Model file for the job. Use its own axes, mm. Face numbers are marked on the shaded views. A direction names the side the tool comes from. Coordinates: 2 decimals unless noted, no trailing zeros. Order: outer loops, then holes, each group sorted by start corner. A loop starts at its lowest first (then second) coordinate and runs counter-clockwise, first axis right, second up. Notation, with made-up numbers: (-11.5, -19.5) - (42.5, -19.5) arc R25 ccw to (42.5, 17.5) - close; hole circle Ø10 at (73.5, 64.5). An arc over 180 degrees is marked (long way). Put each result on its own line as item: value. Start each with the question number.
```python
from build123d import *
from build123d.topology import SkipClean

# Parameters (mm, degrees)
SKETCH_1_W                = 76.6
SKETCH_1_H                = 23.8
EXTRUDE_1_DEPTH           = 31.899999991
HOLE_WIZARD_M4_1_D        = 3.3
HOLE_WIZARD_M4_1_DEPTH    = 10.1
HOLE_WIZARD_M4_1_TIP      = 0.991420021
SKETCH_5_W                = 23.8
SKETCH_5_H                = 2.281370048
EXTRUDE_2_DEPTH           = 2.994
SKETCH_6_W                = 76.6
SKETCH_6_H                = 2.281370048
EXTRUDE_3_DEPTH           = 2.944
CUT_EXTRUDE_START         = -2.994
SKETCH_7_W                = 26.992148155
SKETCH_7_H                = 47.339562986
CUT_EXTRUDE_1_DEPTH       = 2.994
EXTRUDE_4_DEPTH           = 10
HOLE_WIZARD_3_D           = 6.6
HOLE_WIZARD_3_CBORE_D     = 11
HOLE_WIZARD_3_CBORE_DEPTH = 6.8
SKETCH_21_R               = 3.3
CUT_EXTRUDE_6_DEPTH       = 67.034934903
MM_2_D                    = 4
MM_2_DEPTH                = 5
MM_2_TIP                  = 1.201721238
CUT_EXTRUDE_7_DEPTH       = 5
SKETCH_26_W               = 46.053862543
SKETCH_26_H               = 10
CUT_EXTRUDE_8_DEPTH       = 76.924939501
CUT_EXTRUDE_9_DEPTH       = 67.034934903
SKETCH_29_R               = 1
CUT_EXTRUDE_10_DEPTH      = 2.281370048
EXTRUDE_START             = 4
EXTRUDE_5_DEPTH           = 4
CUT_EXTRUDE_11_DEPTH      = 0.5
EXTRUDE_6_DEPTH           = 0.499988059
CUT_EXTRUDE_12_DEPTH      = 28.181370038
SKETCH_35_W               = 0.334557313
SKETCH_35_H               = 10
CUT_EXTRUDE_13_DEPTH      = 100.522674932
CHAMFER_1_SIZE            = 2
HOLE_WIZARD_4_D           = 4.5
HOLE_WIZARD_4_CBORE_D     = 8
HOLE_WIZARD_4_CBORE_DEPTH = 25
CUT_EXTRUDE_14_DEPTH      = 67.269104052
CUT_EXTRUDE_15_DEPTH      = 6.281370048
EXTRUDE_9_DEPTH           = 0.006


with BuildPart() as part:
    # 草图1 → 凸台-拉伸1 (new body)
    with BuildSketch(Plane(origin=(0, 0, 0), x_dir=(1, 0, 0), z_dir=(0, 1, 0))):
        Rectangle(SKETCH_1_W, SKETCH_1_H)
    extrude(amount=-EXTRUDE_1_DEPTH)

    # M4 螺纹孔1
    with Locations(Plane(origin=(0, 0, -5.4), x_dir=(0, 0, 1), z_dir=(0, 1, 0))):
        with Locations((0, 0)):
            Hole(HOLE_WIZARD_M4_1_D / 2, depth=HOLE_WIZARD_M4_1_DEPTH)
            with Locations((0, 0, -(HOLE_WIZARD_M4_1_DEPTH + HOLE_WIZARD_M4_1_TIP / 2))):  # 118° drill point
                Cone(0, HOLE_WIZARD_M4_1_D / 2, HOLE_WIZARD_M4_1_TIP, mode=Mode.SUBTRACT)

    # 草图5 → 凸台-拉伸2 (add)
    with BuildSketch(Plane.ZY.offset(38.3)):
        with Locations((0, 1.140685024)):
            Rectangle(SKETCH_5_W, SKETCH_5_H)
    extrude(amount=-EXTRUDE_2_DEPTH)

    # 草图6 → 凸台-拉伸3 (add)
    with BuildSketch(Plane(origin=(0, 0, -11.9), x_dir=(-1, 0, 0), z_dir=(0, 0, -1))):
        with Locations((0, 1.140685024)):
            Rectangle(SKETCH_6_W, SKETCH_6_H)
    extrude(amount=-EXTRUDE_3_DEPTH)

    # 草图7 → 切除-拉伸1 (cut)
    with BuildSketch(Plane(origin=(38.3, 0, 0), x_dir=(0, 0, -1), z_dir=(1, 0, 0)).offset(CUT_EXTRUDE_START)):
        with Locations((-1.596074077, -8.230218498)):
            Rectangle(SKETCH_7_W, SKETCH_7_H)
    extrude(amount=CUT_EXTRUDE_1_DEPTH, mode=Mode.SUBTRACT)

    # 草图9 → 大小mm 暗销孔1 (revolve, cut)
    with BuildSketch(Plane(origin=(17.4625, 0, -4.384), x_dir=(0, 0, 1), z_dir=(1, 0, 0))):
        Polygon((0, 0), (0, 5.96137699), (1.6, 5), (1.6, 0), align=None)
    mm_1 = revolve(axis=Axis((17.4625, 6.35, -4.384), (0, -1, 0)), mode=Mode.SUBTRACT)

    # 镜向3: 大小mm 暗销孔1 across plane
    add(mm_1.mirror(Plane(origin=(0, 0, 0), x_dir=(0, 0, 1), z_dir=(1, 0, 0))), mode=Mode.SUBTRACT)

    # 草图16 → 凸台-拉伸4 (add)
    with BuildSketch(Plane.XZ.offset(31.899999991)):
        Polygon((-38.3, 6.921881597), (-55.247298311, -11.9), (-38.3, -11.9), align=None)
        Polygon((-33.817682057, 11.9), (-20.311621392, 26.9), (35.306, 26.9), (35.306, 11.9), align=None)
    extrude(amount=-EXTRUDE_4_DEPTH)

    # 打孔尺寸(%根据)内六角圆柱头螺钉的类型3 (through all)
    with Locations(Plane(origin=(-14.255841028, -21.899999991, 19.4), x_dir=(1, 0, 0), z_dir=(0, 1, 0))):
        with Locations((0, 0), (15, 0), (35, 0)):
            CounterBoreHole(HOLE_WIZARD_3_D / 2, HOLE_WIZARD_3_CBORE_D / 2, HOLE_WIZARD_3_CBORE_DEPTH)

    # 草图21 → 切除-拉伸6 (cut, through all)
    with BuildSketch(Plane(origin=(0, -21.899999991, 0), x_dir=(1, 0, 0), z_dir=(0, 1, 0))):
        with Locations(Location((-44.3, 5.9, 0), (0, 0, 180))):
            Circle(SKETCH_21_R)
    extrude(amount=-CUT_EXTRUDE_6_DEPTH, mode=Mode.SUBTRACT)

    # 大小mm 暗销孔2
    with Locations(Plane(origin=(10.744158972, -31.899999991, 9.4), x_dir=(0, 0, -1), z_dir=(0, -1, 0))):
        with Locations((0, 0)):
            Hole(MM_2_D / 2, depth=MM_2_DEPTH)
            with Locations((0, 0, -(MM_2_DEPTH + MM_2_TIP / 2))):  # 118° drill point
                Cone(0, MM_2_D / 2, MM_2_TIP, mode=Mode.SUBTRACT)

    # 草图25 → 切除-拉伸7 (cut)
    with BuildSketch(Plane.XZ.offset(31.899999991)):
        with BuildLine():
            Line((-9.755841028, 11.4), (-8.755841028, 11.4))
            ThreePointArc((-8.755841028, 11.4), (-6.755841028, 9.4), (-8.755841028, 7.4))
            Line((-8.755841028, 7.4), (-9.755841028, 7.4))
            ThreePointArc((-9.755841028, 7.4), (-11.755841028, 9.4), (-9.755841028, 11.4))
        make_face()
    extrude(amount=-CUT_EXTRUDE_7_DEPTH, mode=Mode.SUBTRACT)

    # 草图26 → 切除-拉伸8 (cut, through all)
    with BuildSketch(Plane(origin=(-24.593701474, 0, 22.144268272), x_dir=(0.6691306063588817, 0, 0.7431448254773731), z_dir=(-0.7431448254773731, 0, 0.6691306063588817))):
        with Locations((-11.827706241, -26.899999991)):
            Rectangle(SKETCH_26_W, SKETCH_26_H)
    extrude(amount=CUT_EXTRUDE_8_DEPTH, mode=Mode.SUBTRACT)

    # 草图27 → 切除-拉伸9 (cut, through all)
    with BuildSketch(Plane.XZ.offset(21.899999991)):
        Polygon((-38.3, 6.921881597), (-33.817682057, 11.9), (-38.3, 11.9), align=None)
    extrude(amount=-CUT_EXTRUDE_9_DEPTH, mode=Mode.SUBTRACT)

    # 草图29 → 切除-拉伸10 (cut)
    with BuildSketch(Plane(origin=(0, 2.281370048, 0), x_dir=(1, 0, 0), z_dir=(0, 1, 0))):
        with Locations((-35.306, 8.956)):
            Circle(SKETCH_29_R)
    extrude(amount=-CUT_EXTRUDE_10_DEPTH, mode=Mode.SUBTRACT)

    # 草图31 → 凸台-拉伸5 (add)
    with SkipClean():  # the faces are left unmerged after this step: merging them gives an invalid solid
        with BuildSketch(Plane(origin=(0, 2.281370048, 0), x_dir=(1, 0, 0), z_dir=(0, 1, 0)).offset(EXTRUDE_START)):
            with BuildLine():
                Line((-34.306, 8.956), (35.306, 8.956))
                Line((35.306, 8.956), (35.306, 11.9))
                Line((35.306, 11.9), (-38.3, 11.9))
                Line((-38.3, 11.9), (-38.3, -6.921881597))
                Line((-38.3, -6.921881597), (-35.306, -10.247055466))
                Line((-35.306, -10.247055466), (-35.306, 7.956))
                ThreePointArc((-35.306, 7.956), (-36.013106781, 9.663106781), (-34.306, 8.956))
            make_face()
        extrude(amount=-EXTRUDE_5_DEPTH)

    # 草图32 → 切除-拉伸11 (cut)
    with SkipClean():  # the faces are left unmerged after this step: merging them gives an invalid solid
        with BuildSketch(Plane(origin=(-24.593701474, 0, 22.144268272), x_dir=(0.6691306063588817, 0, 0.7431448254773731), z_dir=(-0.7431448254773731, 0, 0.6691306063588817))):
            Polygon((-23.813531784, -21.899999991), (-45.811081642, -21.899999991), (-45.811081642, -31.899999991), (7.49870663, -31.899999991), (7.49870663, -21.899999991), (-11.951824765, -21.899999991), (-11.951824765, 0), (-16.009278942, 0), (-16.009278942, 6.281370048), (-23.813531784, 6.281370048), align=None)
        extrude(amount=-CUT_EXTRUDE_11_DEPTH, mode=Mode.SUBTRACT)

    # 草图33 → 凸台-拉伸6 (add)
    with SkipClean():  # the faces are left unmerged after this step: merging them gives an invalid solid
        with BuildSketch(Plane(origin=(-24.222129061, 0, 21.809702968), x_dir=(0.6691306063588818, 0, 0.743144825477373), z_dir=(-0.743144825477373, 0, 0.6691306063588818))):
            Polygon((-45.36087962, -21.899999991), (-45.36087962, -31.899999991), (6.849670289, -31.899999991), (6.849670289, -21.899999991), (-13.334820655, -21.899999991), (-13.334820655, 0), (-16.564585199, 0), (-16.564585199, 6.281370048), (-21.03904799, 6.281370048), (-21.03904799, -21.899999991), align=None)
        extrude(amount=EXTRUDE_6_DEPTH)

    # 草图34 → 切除-拉伸12 (cut)
    with SkipClean():  # the faces are left unmerged after this step: merging them gives an invalid solid
        with BuildSketch(Plane(origin=(0, 6.281370048, 0), x_dir=(1, 0, 0), z_dir=(0, 1, 0))):
            Polygon((-38.3, -6.174643322), (-38.3, -6.921863751), (-38.671563539, -6.509200635), align=None)
            Polygon((-33.144865692, -11.9), (-33.817665989, -11.9), (-33.516429231, -12.234557313), align=None)
        extrude(amount=-CUT_EXTRUDE_12_DEPTH, mode=Mode.SUBTRACT)

    # 草图35 → 切除-拉伸13 (cut, through all)
    with SkipClean():  # the faces are left unmerged after this step: merging them gives an invalid solid
        with BuildSketch(Plane(origin=(35.306, 0, 0), x_dir=(0, 0, -1), z_dir=(1, 0, 0))):
            with Locations((-27.067278657, -26.899999991)):
                Rectangle(SKETCH_35_W, SKETCH_35_H)
        extrude(amount=-CUT_EXTRUDE_13_DEPTH, mode=Mode.SUBTRACT)

    # 倒角1
    # the kernel refuses this chamfer: 2 mm, written as the material it takes off along each edge
    with BuildSketch(Plane(origin=(-54.946045485, -16.756634015, -11.565442687), x_dir=(0.7244655223975927, 0, -0.6893110378176047), z_dir=(0, -1, 0))) as chamfer_1_piece_1:
        Polygon((CHAMFER_1_SIZE * 0.999621916911, CHAMFER_1_SIZE * 0.0274958766106), (-CHAMFER_1_SIZE * 0.0274958766106, CHAMFER_1_SIZE * 0.999621916911), (0, 0), align=None)
    extrude(amount=20.286731952, mode=Mode.SUBTRACT)
    with BuildSketch(Plane(origin=(-35.677563539, 0, 9.834374504), x_dir=(-0.6893110378176056, 0, -0.7244655223975918), z_dir=(0, 1, 0))) as chamfer_1_piece_2:
        Polygon((CHAMFER_1_SIZE * 0.999621916911, -CHAMFER_1_SIZE * 0.0274958766106), (-CHAMFER_1_SIZE * 0.0274958766106, -CHAMFER_1_SIZE * 0.999621916911), (0, 0), align=None)
    extrude(amount=11.424736024, mode=Mode.SUBTRACT)

    # 打孔尺寸(%根据)内六角圆柱头螺钉的类型4 (through all)
    with Locations(Plane(origin=(12.5, -31.899999991, -4.384), x_dir=(0, 0, -1), z_dir=(0, -1, 0))):
        with Locations((0, 0)):
            hole_wizard_4 = CounterBoreHole(HOLE_WIZARD_4_D / 2, HOLE_WIZARD_4_CBORE_D / 2, HOLE_WIZARD_4_CBORE_DEPTH)

    # 镜向4: 打孔尺寸(%根据)内六角圆柱头螺钉的类型4 across plane
    add(hole_wizard_4.mirror(Plane(origin=(0, 0, 0), x_dir=(0, 0, 1), z_dir=(1, 0, 0))), mode=Mode.SUBTRACT)

    # 草图39 → 切除-拉伸14 (cut, through all)
    with BuildSketch(Plane(origin=(0, -21.899999991, 0), x_dir=(1, 0, 0), z_dir=(0, 1, 0))):
        Polygon((-53.512357727, 11.9), (-53.512357727, 9.97317112), (-53.607784272, 10.079153036), align=None)
    extrude(amount=-CUT_EXTRUDE_14_DEPTH, mode=Mode.SUBTRACT)

    # 草图40 → 切除-拉伸15 (cut)
    with BuildSketch(Plane(origin=(0, 6.281370048, 0), x_dir=(1, 0, 0), z_dir=(0, 1, 0))):
        Polygon((-38.3, -6.921863751), (-35.306, -6.921863751), (-35.306, -8.437692972), (-37.015824752, -8.348084853), align=None)
    extrude(amount=-CUT_EXTRUDE_15_DEPTH, mode=Mode.SUBTRACT)

    # 草图42 → 凸台-拉伸9 (add)
    with BuildSketch(Plane.ZY.offset(38.3)):
        Polygon((-11.9, -21.899999991), (6.921863751, -21.899999991), (6.921863751, 0), (6.921863751, 6.281370048), (-11.9, 6.281370048), align=None)
    extrude(amount=EXTRUDE_9_DEPTH)


solid = part.part
```
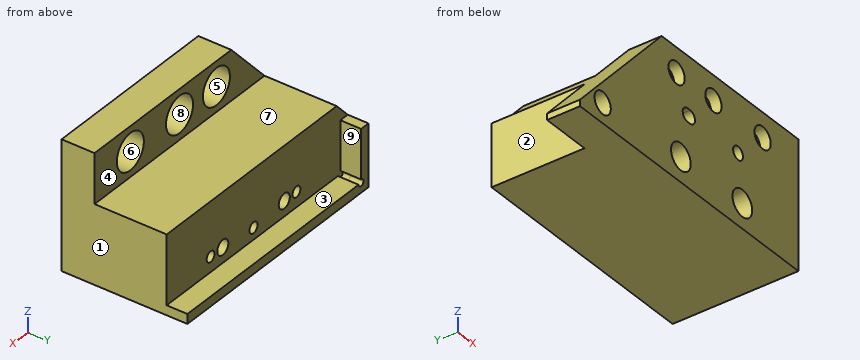
Item 1: Slice it at A-A, the plane y = -21. Give the number of separate pieces and of enclosed holes in the cut face, plus the area to 3 significant figures.
Item 2: Pull direction X, two halves, no side cores. Call the marked faces 6, 7, 8 and 9: pulls with the +X half, pulls with the -X half, needs draft (parallel to the pull), parting line crosses it, or undercut.
Item 3: Wall check: line 1 along X through (y, z) = (-24.5, -6); line 2 along X through (y, z) = (-23.75, 19.4); line 3 along Z through (x, y) = (27, -17.5). Give the ranges that are in metal, low to high.
Item 4: Slice it at C-C, the plane x = -44.3. Give the cut face in (y, z).
Item 5: Slice it at B-B, the plane x = 30.5. Give the cut face in (y, z).
Item 6: Flat gauge pins, fed straight in: pin 1 Ø12 at (x, z) = (20.5, 17) entering from +Y; pin 2 Ø10 at (x, z) = (-15.5, 21) entering from -Y; pin 3 Ø12 at (x, y) = (-26.5, 1.5) entering from +Z; pin 4 Ø6 at (x, z) = (-14.26, 19.4) entering from -Y. Where does each tip first touch, or does it go through?
Item 7: 3-axis set-ups, long thin cutter, end or side, ignore diameter. For the marked faces 1, 2, 3, 4 and 5: which of +Z, -Z, +X, -X, +Y, -Y reach the whole face in a straight line?
Here are the results:
1. separate pieces: 1
1. enclosed holes: 2
1. area: 1,640 mm^2
2. face 6: undercut
2. face 7: needs draft
2. face 8: undercut
2. face 9: pulls with the +X half
3. line 1: x = -49.93 to -47.6, -41 to -16.16, -8.84 to 8.84, 16.16 to 35.31
3. line 2: x = -27.06 to -19.76, -8.76 to -4.76, 6.24 to 15.24, 26.24 to 35.31
3. line 3: z = -11.9 to 11.9
4. outline: (-31.9, -11.9) - (-21.9, -11.9) - (-21.9, -9.2) - (-31.9, -9.2) - close; (-31.9, -2.6) - (-21.9, -2.6) - (-21.9, 0.26) - (-31.9, 0.26) - close
5. outline: (-31.9, -11.9) - (6.28, -11.9) - (6.28, -8.96) - (0, -8.96) - (0, 11.9) - (-21.9, 11.9) - (-21.9, 26.9) - (-31.9, 26.9) - close
6. pin 1: stops at y = 0
6. pin 2: stops at y = -31.9
6. pin 3: stops at z = 11.9
6. pin 4: passes through
7. face 1: +Z, -Z, +X, +Y, -Y
7. face 2: +Z, -Z, -X, +Y
7. face 3: +Z, +X, +Y
7. face 4: +Z, +X, -X, +Y
7. face 5: +Y
